Geometry: final body of the model. Coordinates: model frame, mm. Round coordinates to 2 decimals unless told otherwise and drop trailing zeros. Loops run counter-clockwise (first coordinate to the right, second up) from the corner with the lowest first, then second, coordinate; pieces in that order, holes last. Notation, with made-up numbers: M 60.25,84.25 L 98.25,84.25 A11 cw 98.25,100.25 Z; hole C 66.5,26 d11. An arc over 180 degrees is marked long. Return JSON: item names as keys, results as strings.
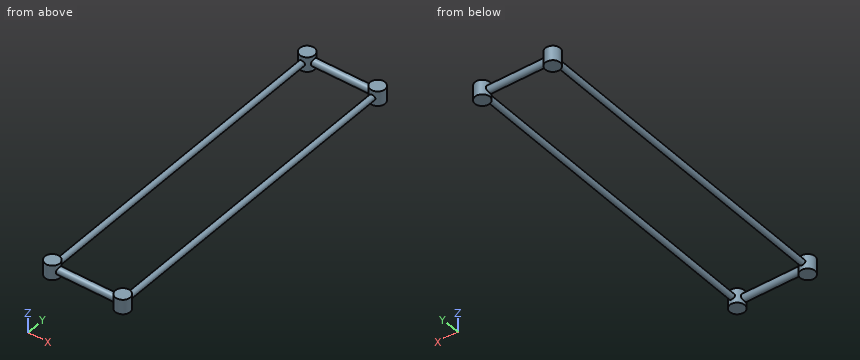
from build123d import *

# Parameters (mm, degrees)
SKETCH1_R                = 5
BOSS_EXTRUDE1_DEPTH      = 80
BOSS_EXTRUDE2_DEPTH      = 10
BOSS_EXTRUDE2_DEPTH_BACK = 10
SKETCH2_R                = 10
SKETCH3_R                = 3.98820793
BOSS_EXTRUDE3_DEPTH      = 448


with BuildPart() as part:
    # Sketch1 → Boss-Extrude1 (new body)
    with BuildSketch(Plane(origin=(0, 0, 0), x_dir=(0, 0, -1), z_dir=(1, 0, 0))):
        Circle(SKETCH1_R)
    extrude(amount=BOSS_EXTRUDE1_DEPTH)


with BuildPart() as body_2:
    # Sketch2 → Boss-Extrude2 (new, two sides: drawn at the far end of the back side and taken through both)
    with BuildSketch(Plane.XY.offset(-BOSS_EXTRUDE2_DEPTH_BACK)):
        with Locations((-7.666034923, 0)):
            Circle(SKETCH2_R)
    extrude(amount=BOSS_EXTRUDE2_DEPTH + BOSS_EXTRUDE2_DEPTH_BACK)

    # Sketch3 → Boss-Extrude3 (add)
    with BuildSketch(Plane(origin=(0, 0, 0), x_dir=(1, 0, 0), z_dir=(0, 1, 0))):
        with Locations(Location((-7.666034923, 0, 0), (0, 0, 270))):
            Circle(SKETCH3_R)
    extrude(amount=-BOSS_EXTRUDE3_DEPTH)


with BuildPart() as body_3:
    # Mirror1: mirrored copy
    add(part.part.mirror(Plane.ZX.offset(-224)))


with BuildPart() as body_4:
    # Mirror1 2: mirrored copy
    add(body_2.part.mirror(Plane.ZX.offset(-224)))


with BuildPart() as body_5:
    # Mirror2: mirrored copy
    add(part.part.mirror(Plane.ZY.offset(-40)))


with BuildPart() as body_6:
    # Mirror2 2: mirrored copy
    add(body_3.part.mirror(Plane.ZY.offset(-40)))


with BuildPart() as body_7:
    # Mirror2 3: mirrored copy
    add(body_4.part.mirror(Plane.ZY.offset(-40)))


with BuildPart() as body_8:
    # Mirror2 4: mirrored copy
    add(body_2.part.mirror(Plane.ZY.offset(-40)))


with BuildPart() as body_7_1:
    add(body_7.part)

    # Combine1: union part, body 8, body 5, body 2, body 3, body 6, body 4
    add(part.part)
    add(body_8.part)
    add(body_5.part)
    add(body_2.part)
    add(body_3.part)
    add(body_6.part)
    add(body_4.part)


solid = body_7_1.part
Q1. Section query D-D (y = -116). Output: boundary loops of the cut face in (x, z).
Determined:
{"outline": "C -7.67,0 d7.98; C 87.67,0 d7.98"}
Q2. Material intervals for L1, parallel to X at y = -48, z = 0; L2, parallel to Y at x = 4, z = 0; L3, parallel to Y at x = -7, z = -0.25, sorted ascending.
Determined:
{"L1": "x = -11.65 to -3.68, 83.68 to 91.65", "L2": "y = -453 to -443, -5 to 5", "L3": "y = -457.98 to 9.98"}
Q3. Pin query (flat end, axial travel): pin 1 (8 mm diameter, centred on x = 32, z = -7.5, fed in from +Y); pin 2 (4 mm diameter, centred on x = 83, z = -1, fed in from -Y); pin 3 (2 mm diameter, centred on x = 40.5, z = 5, fed in from +Y). Return the tip coordinate at first contact, or that it passes through.
Determined:
{"pin 1": "stops at y = 3.57", "pin 2": "stops at y = -457.64", "pin 3": "stops at y = 3"}
Q4. Section query A-A (z = 0). Output: boundary loops of the cut face in (x, y), plus the area to 3 significant figures.
Determined:
{"outline": "M -11.65,-438.83 A10 ccw long 0.99,-453 L 79.01,-453 A10 ccw long 91.65,-438.83 L 91.65,-9.17 A10 ccw long 79.01,5 L 0.99,5 A10 ccw long -11.65,-9.17 Z; hole M -3.68,-438.83 A10 cw 0.99,-443 L 79.01,-443 A10 cw 83.68,-438.83 L 83.68,-9.17 A10 cw 79.01,-5 L 0.99,-5 A10 cw -3.68,-9.17 Z", "area": "9,620 mm^2"}
Q5. Section query B-B (x = 35.5). Output: boundary loops of the cut face in (y, z).
Determined:
{"outline": "C -448,0 d10; C 0,0 d10"}
Q6. Section query C-C (y = -448). Output: boundary loops of the cut face in (x, z), plus the area to 3 significant figures.
Determined:
{"outline": "M -17.67,-10 L 2.33,-10 L 2.33,-5 L 77.67,-5 L 77.67,-10 L 97.67,-10 L 97.67,10 L 77.67,10 L 77.67,5 L 2.33,5 L 2.33,10 L -17.67,10 Z", "area": "1,550 mm^2"}
